Can you work these out from the model? Positions are in its coordinate system, mm. Coordinates: 2 decimals unless noted, no trailing zeros. Loops run counter-clockwise (first coordinate to the right, second up) from the corner with the lowest first, then second, coordinate; pieces in that order, holes last. Notation, with made-up numbers: (-31, 13.25) -> (-14, 13.25) arc R20 cw to (-14, 50.25) -> close; hole circle Ø9 at (34.25, 14.5). An arc over 180 degrees is marked (long way). Put each result on its own line as item: value. Start each with the question number.
Item 1: If we section it at C-C on x = 67.5: Please give me the cut outline in (y, z).
Item 2: Please list where these lines run through material, in increasing order: L1, parallel to Z at x = 38, y = -2.25; L2, parallel to Z at x = 67, y = -0.55 (3 decimals); L3, parallel to X at y = -0.8, z = 9. Write a range as from..to.
Item 3: If we section it at B-B on x = 85: Please give me the cut outline in (y, z), plus the area to 3 significant figures.
Item 4: If we section it at A-A on z = 87.5: Please give me the cut outline in (x, y), plus the area to 3 significant figures.
Item 5: If we section it at D-D on y = -0.9: State how many separate pieces and enclosed holes the cut face has, plus the area to 3 significant figures.
Item 6: Will these pins go through, and if not, where does the flat tip stop? P1, Ø1.5, axis at x = 89, y = -2, coming from the +Z side; P2, Ø1.5, axis at x = 37.5, y = -1.5, coming from the +Z side.
```python
from build123d import *

# Parameters (mm, degrees)
F1_DEPTH = 3


with BuildPart() as f1:
    # F0 (on Front) → F1 (new body)
    with BuildSketch(Plane.XZ):
        with BuildLine():
            ThreePointArc((0, 4), (1.171573, 1.171573), (4, 0))
            Line((4, 0), (96, 0))
            ThreePointArc((96, 0), (98.828427, 1.171573), (100, 4))
            Line((100, 4), (100, 96))
            ThreePointArc((100, 96), (98.828427, 98.828427), (96, 100))
            Line((96, 100), (70, 100))
            ThreePointArc((70, 100), (62.928932, 102.928932), (60, 110))
            Line((60, 110), (40, 110))
            ThreePointArc((40, 110), (37.071068, 102.928932), (30, 100))
            Line((30, 100), (4, 100))
            ThreePointArc((4, 100), (1.171573, 98.828427), (0, 96))
            Line((0, 96), (0, 4))
        make_face()
        with BuildLine():
            Line((92, 4), (8, 4))
            ThreePointArc((8, 4), (5.171573, 5.171573), (4, 8))
            Line((4, 8), (4, 26.62902))
            ThreePointArc((4, 26.62902), (4.687882, 28.138439), (6.278346, 28.609556))
            Line((6.278346, 28.609556), (94.278346, 16.241963))
            ThreePointArc((94.278346, 16.241963), (95.509419, 15.573545), (96, 14.261427))
            Line((96, 14.261427), (96, 8))
            ThreePointArc((96, 8), (94.828427, 5.171573), (92, 4))
        make_face(mode=Mode.SUBTRACT)
        with BuildLine():
            Line((93.721654, 20.359511), (5.721654, 32.727104))
            ThreePointArc((5.721654, 32.727104), (4.490581, 33.395523), (4, 34.707641))
            Line((4, 34.707641), (4, 51.929757))
            Line((4, 51.929757), (94.278346, 39.241963))
            ThreePointArc((94.278346, 39.241963), (95.509419, 38.573545), (96, 37.261427))
            Line((96, 37.261427), (96, 22.340047))
            ThreePointArc((96, 22.340047), (95.312118, 20.830628), (93.721654, 20.359511))
        make_face(mode=Mode.SUBTRACT)
        with BuildLine():
            Line((93.721654, 43.359511), (5.721654, 55.727104))
            ThreePointArc((5.721654, 55.727104), (4.490581, 56.395523), (4, 57.707641))
            Line((4, 57.707641), (4, 72.62902))
            ThreePointArc((4, 72.62902), (4.687882, 74.138439), (6.278346, 74.609556))
            Line((6.278346, 74.609556), (94.278346, 62.241963))
            ThreePointArc((94.278346, 62.241963), (95.509419, 61.573545), (96, 60.261427))
            Line((96, 60.261427), (96, 45.340047))
            ThreePointArc((96, 45.340047), (95.312118, 43.830628), (93.721654, 43.359511))
        make_face(mode=Mode.SUBTRACT)
        with BuildLine():
            ThreePointArc((4, 92), (5.171573, 94.828427), (8, 96))
            Line((8, 96), (92, 96))
            ThreePointArc((92, 96), (94.828427, 94.828427), (96, 92))
            Line((96, 92), (96, 68.340047))
            ThreePointArc((96, 68.340047), (95.312118, 66.830628), (93.721654, 66.359511))
            Line((93.721654, 66.359511), (5.721654, 78.727104))
            ThreePointArc((5.721654, 78.727104), (4.490581, 79.395523), (4, 80.707641))
            Line((4, 80.707641), (4, 92))
        make_face(mode=Mode.SUBTRACT)
    extrude(amount=F1_DEPTH)


solid = f1.part
```
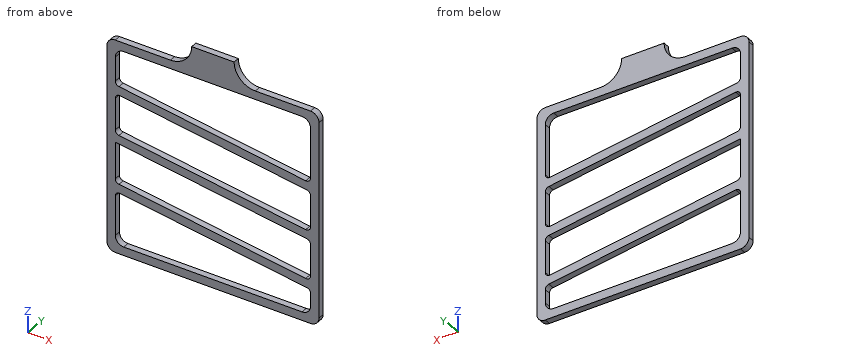
Solutions:
1. outline: (-3, 0) -> (0, 0) -> (0, 4) -> (-3, 4) -> close; (-3, 20.01) -> (0, 20.01) -> (0, 24.04) -> (-3, 24.04) -> close; (-3, 43.01) -> (0, 43.01) -> (0, 47.04) -> (-3, 47.04) -> close; (-3, 66.01) -> (0, 66.01) -> (0, 70.04) -> (-3, 70.04) -> close; (-3, 96) -> (0, 96) -> (0, 100.32) -> (-3, 100.32) -> close
2. L1: 0..4, 24.15..28.19, 47.15..51.19, 70.15..74.19, 96..104
2. L2: 0..4, 20.076..24.115, 43.076..47.115, 66.076..70.115, 96..100.461
2. L3: 0..4, 96..100
3. outline: (-3, 0) -> (0, 0) -> (0, 4) -> (-3, 4) -> close; (-3, 17.55) -> (0, 17.55) -> (0, 21.59) -> (-3, 21.59) -> close; (-3, 40.55) -> (0, 40.55) -> (0, 44.59) -> (-3, 44.59) -> close; (-3, 63.55) -> (0, 63.55) -> (0, 67.59) -> (-3, 67.59) -> close; (-3, 96) -> (0, 96) -> (0, 100) -> (-3, 100) -> close
3. area: 60.4 mm^2
4. outline: (0, -3) -> (4, -3) -> (4, 0) -> (0, 0) -> close; (96, -3) -> (100, -3) -> (100, 0) -> (96, 0) -> close
4. area: 24.0 mm^2
5. separate pieces: 1
5. enclosed holes: 4
5. area: 2,900 mm^2
6. P1: z = 100
6. P2: z = 104.35
